Model file for the job. Use its own axes, mm. Face numbers are marked on the shaded views. A direction names the side the tool comes from. Coordinates: 2 decimals unless noted, no trailing zeros. Order: outer loops, then holes, each group sorted by start corner. A loop starts at its lowest first (then second) coordinate and runs counter-clockwise, first axis right, second up. Notation, with made-up numbers: (-37.5, 56) -> (21.5, 56) arc R20 ccw to (21.5, 76) -> close; hole circle Ø1 at (-36.75, 9). An arc over 180 degrees is marked (long way). Use CSV: the item, a comma, the result in double quotes. Start each with the question number.
(1) Tool access for the marked faces 1 and 2: list every direction of +Z, -Z, +X, -X, +Y, -Y with a clear straight run to the whole face (end or side of a thin tool).
(2) Cut at B-B on y = 6.5. Write the cut outline in (x, z).
(3) Cut at C-C on z = -33. Give the number of separate pieces and of enclosed holes in the cut face, plus the area to 3 significant figures.
(4) Pin check, flat tips, straight feed: pin 1 Ø3.5 at (y, z) = (-30, -37) entering from +X; pin 2 Ø3 at (x, z) = (-41, -28) entering from +Y; pin 3 Ø3 at (x, z) = (-48, 65.5) entering from +Y. Stop position of each tip, or through.
(5) Cut at A-A on z = 10. Write the cut outline in (x, y).
(6) Probe L1, parallel to X at y = -10.5, z = 8; L2, parallel to Z at x = -2, y = -4; L3, parallel to Y at x = 73.8, z = -50. List the from-to ranges inside material, lowest first.
(7) Pull direction X, two halves, no side cores. Call the marked faces 3, 4, 5 and 6: pulls with the +X half, pulls with the -X half, needs draft (parallel to the pull), parting line crosses it, or undercut.
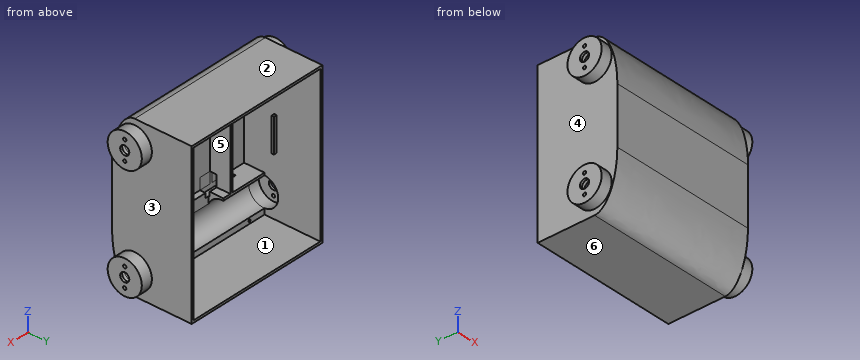
```python
from build123d import *
from build123d.topology import SkipClean

# Parameters (mm, degrees)
EXTRUDE_1_DEPTH          = 35
EXTRUDE_1_DEPTH_BACK     = 35
SKETCH_1_W               = 130
SKETCH_1_H               = 140
CUT_EXTRUDE_1_DEPTH      = 130
SKETCH_3_W               = 126
SKETCH_3_H               = 136
CUT_EXTRUDE_2_DEPTH      = 49
CUT_EXTRUDE_3_DEPTH      = 63
CUT_EXTRUDE_3_DEPTH_BACK = 63
SKETCH_4_R               = 13
SKETCH_8_R               = 15
EXTRUDE_3_DEPTH          = 10
CUT_EXTRUDE_6_DEPTH      = 32
CUT_EXTRUDE_6_DEPTH_BACK = 160
SKETCH_7_R               = 1.4
SKETCH_7_R_2             = 4
CUT_EXTRUDE_7_DEPTH      = 136
CUT_EXTRUDE_7_DEPTH_BACK = 10
SKETCH_9_R               = 13
SKETCH_10_W              = 32
SKETCH_10_H              = 70
CUT_EXTRUDE_8_DEPTH      = 18
SKETCH_11_W              = 58
SKETCH_11_H              = 70.077037206
CUT_EXTRUDE_9_DEPTH      = 18
SKETCH_13_W              = 44
SKETCH_13_H              = 14.961481397
CUT_EXTRUDE_11_DEPTH     = 13
CUT_EXTRUDE_START        = -4
SKETCH_14_W              = 29
SKETCH_14_H              = 6
CUT_EXTRUDE_12_DEPTH     = 14
SKETCH_15_W              = 30
SKETCH_15_H              = 2
EXTRUDE_4_DEPTH          = 2.5
SKETCH_16_R              = 1
CUT_EXTRUDE_13_DEPTH     = 5
MIRROR_6_COPY_1_SKETCH_R = 1
MIRROR_6_COPY_1_DEPTH    = 5


with BuildPart() as part:
    # Sketch 1 → Extrude 1 (new, two sides: drawn at the far end of the back side and taken through both)
    with BuildSketch(Plane(origin=(0, 0, 0), x_dir=(1, 0, 0), z_dir=(0, 1, 0)).offset(-EXTRUDE_1_DEPTH_BACK)):
        Rectangle(SKETCH_1_W, SKETCH_1_H)
    extrude(amount=EXTRUDE_1_DEPTH + EXTRUDE_1_DEPTH_BACK)

    # Sketch 2 → Cut-Extrude 1 (cut)
    with BuildSketch(Plane(origin=(65, 0, 0), x_dir=(0, 0, -1), z_dir=(1, 0, 0))):
        with BuildLine():
            Line((-25, -35), (25, -35))
            add(Edge.make_bspline(
                [(25, -35), (70, -35), (70, -15)],
                knots=[1.570796327, 1.570796327, 1.570796327, 3.141592654, 3.141592654, 3.141592654], degree=2, weights=[1, 0.707106781, 1]))
            Line((70, -15), (70, -40.742443293))
            Line((70, -40.742443293), (-70, -40.742443293))
            Line((-70, -40.742443293), (-70, -15))
            add(Edge.make_bspline(
                [(-70, -15), (-70, -35), (-25, -35)],
                knots=[0, 0, 0, 1.570796327, 1.570796327, 1.570796327], degree=2, weights=[1, 0.707106781, 1]))
        make_face()
    extrude(amount=-CUT_EXTRUDE_1_DEPTH, mode=Mode.SUBTRACT)

    # Sketch 3 → Cut-Extrude 2 (cut)
    with BuildSketch(Plane(origin=(0, 35, 0), x_dir=(1, 0, 0), z_dir=(0, 1, 0))):
        Rectangle(SKETCH_3_W, SKETCH_3_H)
    extrude(amount=-CUT_EXTRUDE_2_DEPTH, mode=Mode.SUBTRACT)

    # Sketch 4 → Cut-Extrude 3 (cut, two sides: drawn at the far end of the back side and taken through both)
    with BuildSketch(Plane(origin=(0, 0, 0), x_dir=(0, 0, -1), z_dir=(1, 0, 0)).offset(-CUT_EXTRUDE_3_DEPTH_BACK)):
        with Locations((-50, -15)):
            Circle(SKETCH_4_R)
        with Locations((50, -15)):
            Circle(SKETCH_4_R)
    extrude(amount=CUT_EXTRUDE_3_DEPTH + CUT_EXTRUDE_3_DEPTH_BACK, mode=Mode.SUBTRACT)

    # Sketch 8 → Extrude 3 (add)
    with BuildSketch(Plane(origin=(65, 0, 0), x_dir=(0, 0, -1), z_dir=(1, 0, 0))):
        with Locations((-50, -15)):
            Circle(SKETCH_8_R)
        with Locations((50, -15)):
            Circle(SKETCH_8_R)
    extrude_3 = extrude(amount=EXTRUDE_3_DEPTH)

    # Mirror 2: Extrude 3 across plane
    add(extrude_3.mirror(Plane(origin=(0, 0, 0), x_dir=(0, 0, 1), z_dir=(1, 0, 0))))

    # Sketch 7 → Cut-Extrude 6 (cut, two sides: drawn at the far end of the back side and taken through both)
    with BuildSketch(Plane(origin=(65, 0, 0), x_dir=(0, 0, -1), z_dir=(1, 0, 0)).offset(-CUT_EXTRUDE_6_DEPTH_BACK)):
        with Locations(Location((-58.5, -15, 0), (0, 0, 180))):
            Circle(SKETCH_7_R)
        with Locations(Location((-50, -15, 0), (0, 0, 180))):
            Circle(SKETCH_7_R_2)
        with Locations(Location((-41.5, -15, 0), (0, 0, 180))):
            Circle(SKETCH_7_R)
        with Locations(Location((41.5, -15, 0), (0, 0, 180))):
            Circle(SKETCH_7_R)
        with Locations(Location((50, -15, 0), (0, 0, 180))):
            Circle(SKETCH_7_R_2)
        with Locations(Location((58.5, -15, 0), (0, 0, 180))):
            Circle(SKETCH_7_R)
    extrude(amount=CUT_EXTRUDE_6_DEPTH + CUT_EXTRUDE_6_DEPTH_BACK, mode=Mode.SUBTRACT)

    # Sketch 9 → Cut-Extrude 7 (cut, two sides: drawn at the far end of the back side and taken through both)
    with SkipClean():  # the faces are left unmerged after this step: merging them gives an invalid solid
        with BuildSketch(Plane.ZY.offset(-63).offset(-CUT_EXTRUDE_7_DEPTH_BACK)):
            with Locations((-50, -15)):
                Circle(SKETCH_9_R)
            with Locations((50, -15)):
                Circle(SKETCH_9_R)
        extrude(amount=CUT_EXTRUDE_7_DEPTH + CUT_EXTRUDE_7_DEPTH_BACK, mode=Mode.SUBTRACT)

    # Sketch 10 → Cut-Extrude 8 (cut)
    with SkipClean():  # the faces are left unmerged after this step: merging them gives an invalid solid
        with BuildSketch(Plane(origin=(0, -14, 0), x_dir=(1, 0, 0), z_dir=(0, 1, 0))):
            with Locations((-47, -0.038518603)):
                Rectangle(SKETCH_10_W, SKETCH_10_H)
            with Locations((47, -0.038518603)):
                Rectangle(SKETCH_10_W, SKETCH_10_H)
        extrude(amount=-CUT_EXTRUDE_8_DEPTH, mode=Mode.SUBTRACT)

    # Sketch 11 → Cut-Extrude 9 (cut)
    with SkipClean():  # the faces are left unmerged after this step: merging them gives an invalid solid
        with BuildSketch(Plane(origin=(0, -14, 0), x_dir=(1, 0, 0), z_dir=(0, 1, 0))):
            Rectangle(SKETCH_11_W, SKETCH_11_H)
        extrude(amount=-CUT_EXTRUDE_9_DEPTH, mode=Mode.SUBTRACT)

    # Sketch 13 → Cut-Extrude 11 (cut)
    with SkipClean():  # the faces are left unmerged after this step: merging them gives an invalid solid
        with BuildSketch(Plane(origin=(0, -14, 0), x_dir=(1, 0, 0), z_dir=(0, 1, 0))):
            with Locations((0, 42.519259301)):
                Rectangle(SKETCH_13_W, SKETCH_13_H)
            with Locations((0, -42.519259301)):
                Rectangle(SKETCH_13_W, SKETCH_13_H)
        extrude(amount=-CUT_EXTRUDE_11_DEPTH, mode=Mode.SUBTRACT)

    # Sketch 14 → Cut-Extrude 12 (cut)
    with SkipClean():  # the faces are left unmerged after this step: merging them gives an invalid solid
        with BuildSketch(Plane.XY.offset(-35.038518603).offset(CUT_EXTRUDE_START)):
            with Locations((-33.5, -29)):
                Rectangle(SKETCH_14_W, SKETCH_14_H)
        cut_extrude_12 = extrude(amount=CUT_EXTRUDE_12_DEPTH, mode=Mode.SUBTRACT)

    # Sketch 15 → Extrude 4 (add)
    with BuildSketch(Plane.ZY.offset(-63)):
        with Locations((0, -4.5)):
            Rectangle(SKETCH_15_W, SKETCH_15_H)
    extrude_4 = extrude(amount=EXTRUDE_4_DEPTH)

    # Mirror 3: Extrude 4 across plane
    add(extrude_4.mirror(Plane(origin=(0, 0, 0), x_dir=(0, 0, 1), z_dir=(1, 0, 0))))

    # Mirror 4: Cut-Extrude 12 across plane
    add(cut_extrude_12.mirror(Plane(origin=(0, 0, 0), x_dir=(0, 0, 1), z_dir=(1, 0, 0))), mode=Mode.SUBTRACT)

    # Sketch 16 → Cut-Extrude 13 (cut)
    with BuildSketch(Plane(origin=(0, -14, 0), x_dir=(1, 0, 0), z_dir=(0, 1, 0))):
        with Locations(Location((-48, 65.501481397, 0), (0, 0, 270))):
            Circle(SKETCH_16_R)
    cut_extrude_13 = extrude(amount=-CUT_EXTRUDE_13_DEPTH, mode=Mode.SUBTRACT)

    # Mirror 5: Cut-Extrude 13 across plane
    add(cut_extrude_13.mirror(Plane.XY), mode=Mode.SUBTRACT)

    # Mirror 6: Cut-Extrude 13 across plane
    add(cut_extrude_13.mirror(Plane(origin=(0, 0, 0), x_dir=(0, 0, 1), z_dir=(1, 0, 0))), mode=Mode.SUBTRACT)

    # Mirror 6 copy 1 sketch → Mirror 6 copy 1 (cut)
    with BuildSketch(Plane(origin=(0, -14, 0), x_dir=(-1, 0, 0), z_dir=(0, 1, 0))):
        with Locations(Location((-48, 65.501481397, 0), (0, 0, 270))):
            Circle(MIRROR_6_COPY_1_SKETCH_R)
    extrude(amount=-MIRROR_6_COPY_1_DEPTH, mode=Mode.SUBTRACT)


solid = part.part
```
Outcome:
1,face 1,"+Y"
1,face 2,"+Z, +X, -X, +Y, -Y"
2,outline,"(-65, -70) -> (65, -70) -> (65, 70) -> (-65, 70) -> close; hole (-63, -68) -> (63, -68) -> (63, 68) -> (-63, 68) -> close"
3,separate pieces,"3"
3,enclosed holes,"0"
3,area,"665 mm2"
4,pin 1,"x = 65"
4,pin 2,"y = -32"
4,pin 3,"y = -14"
5,outline,"(-65, -35) -> (65, -35) -> (65, 35) -> (63, 35) -> (63, -3.5) -> (60.5, -3.5) -> (60.5, -5.5) -> (63, -5.5) -> (63, -32) -> (31, -32) -> (31, -14) -> (29, -14) -> (29, -32) -> (-29, -32) -> (-29, -14) -> (-31, -14) -> (-31, -32) -> (-63, -32) -> (-63, -5.5) -> (-60.5, -5.5) -> (-60.5, -3.5) -> (-63, -3.5) -> (-63, 35) -> (-65, 35) -> close"
6,L1,"-65 to -63, 63 to 65"
6,L2,"-70 to -68, 68 to 70"
6,L3,"-30 to -19, -11 to 0"
7,face 3,"pulls with the +X half"
7,face 4,"pulls with the -X half"
7,face 5,"undercut"
7,face 6,"needs draft"
